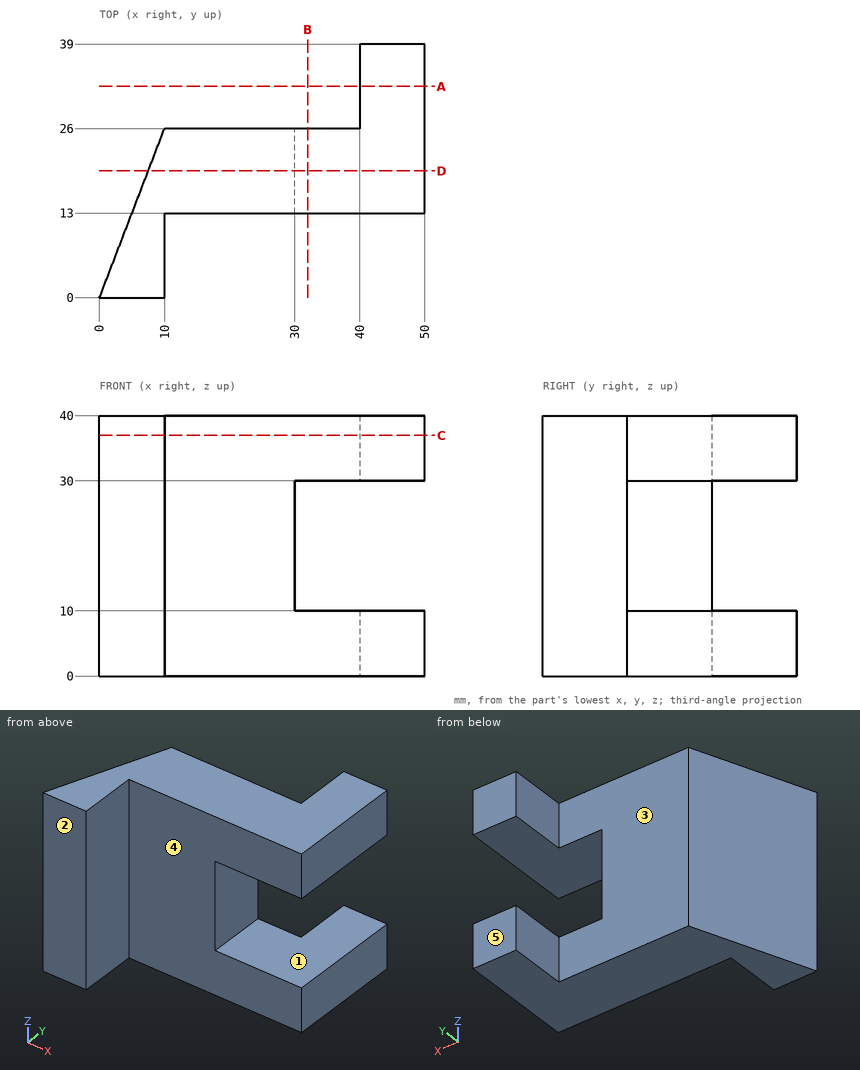
Input: dimensioned drawing with shaded views. Units: mm. Origin: part minimum x, y, z. A direction names the side the tool comes from. Round coordinates to 2 decimals unless told otherwise and drop trailing zeros. Write each loop counter-clockwise with the first axis right and the second up, starting at its lowest first coordinate (ties: lowest second). Pieces come first, ordered by that corner, then holes. Notation, with made-up numbers: (-17, -0.5) - (0, -0.5) arc R27 cw to (0, 30.5) - close; hole circle Ø9 at (-28.5, 55.5). An arc over 180 degrees is marked (long way). Write item = value, one per line.
(1) Section query A-A on y = 32.5. Output: boundary loops of the cut face in (x, z), then the cut area to 3 significant figures.
Geometry check:
outline = (40, 0) - (50, 0) - (50, 10) - (40, 10) - close; (40, 30) - (50, 30) - (50, 40) - (40, 40) - close
area = 200 mm^2
(2) Material intervals for probe 1 along Z at (x, y) = (31.5, 25); probe 2 along Y at (x, z) = (37, 4); probe 3 along Y at (x, z) = (47, 9), sorted ascending.
Geometry check:
probe_1 = 0 to 10, 30 to 40
probe_2 = 13 to 26
probe_3 = 13 to 39
(3) Contact query for flat-ended pins moving along their axis: pin 1 Ø8 at (x, y) = (19, 7) entering from -Z; pin 2 Ø5 at (y, z) = (35.5, 5.5) entering from -X; pin 3 Ø1 at (y, z) = (10, 24.5) entering from +X; pin 4 Ø5 at (x, z) = (36.5, 29.5) entering from -Y. Output: stop coordinate, or through.
Geometry check:
pin_1 = through
pin_2 = 40
pin_3 = 10
pin_4 = 13
(4) Access query for the marked faces 1, 2, 3, 4 and 5. Directions: +Z, -Z, +X, -X, +Y, -Y. A direction counts if a zero-diameter tool reaches every point of the face in a straight line with its end or side. Return the directions, or none.
Geometry check:
face_1 = +X, +Y, -Y
face_2 = +Z, -Z, +X, -X, -Y
face_3 = +Z, -Z, -X, +Y
face_4 = +Z, -Z, +X, -Y
face_5 = +Z, -Z, +X, -X, +Y
(5) Section query B-B on x = 32. Output: boundary loops of the cut face in (y, z).
Geometry check:
outline = (13, 0) - (26, 0) - (26, 10) - (13, 10) - close; (13, 30) - (26, 30) - (26, 40) - (13, 40) - close
(6) Section query C-C on z = 37. Output: boundary loops of the cut face in (x, y), then the cut area to 3 significant figures.
Geometry check:
outline = (0, 0) - (10, 0) - (10, 13) - (50, 13) - (50, 39) - (40, 39) - (40, 26) - (10, 26) - close
area = 780 mm^2
(7) Section query D-D on y = 19.5. Output: boundary loops of the cut face in (x, z), then the cut area to 3 significant figures.
Geometry check:
outline = (7.5, 0) - (50, 0) - (50, 10) - (30, 10) - (30, 30) - (50, 30) - (50, 40) - (7.5, 40) - close
area = 1,300 mm^2
